Answer from the drawing. Dimensions are ordinates in mm from the lowest x, y and z of the part. Coordinates: 2 decimals unless noted, no trailing zeros. Write each loop counter-clockwise with the first axis right and the second up, starting at its lowest first coordinate (ties: lowest second). Pieces come first, ordered by that corner, then holes.
1) Each of these flat-tipped pins is pushed along its axis until it touches: pin 1 Ø1.6 at (y, z) = (1.5, 9.5) entering from -X; pin 2 Ø5 at (x, z) = (23, 21) entering from +Y; pin 3 Ø1 at (y, z) = (1.5, 8.5) entering from +X; pin 4 Ø0.6 at (x, y) = (45.5, 0.5) entering from -Z. Where does it stop, or does it pass through?
2) The part is cut by section A-A (z = 37). Determine the outline of the cut face in (x, y), then the cut area to 3 significant figures.
3) The part is cut by section C-C (y = 6). Determine the outline of the cut face in (x, z).
4) The part is cut by section B-B (x = 12.5). Determine the outline of the cut face in (y, z).
5) Find the intervals of material crossed by line 1 (Z direction, x = 6.5, y = 1.75); line 2 (Y direction, x = 50.5, z = 51), in increasing order.
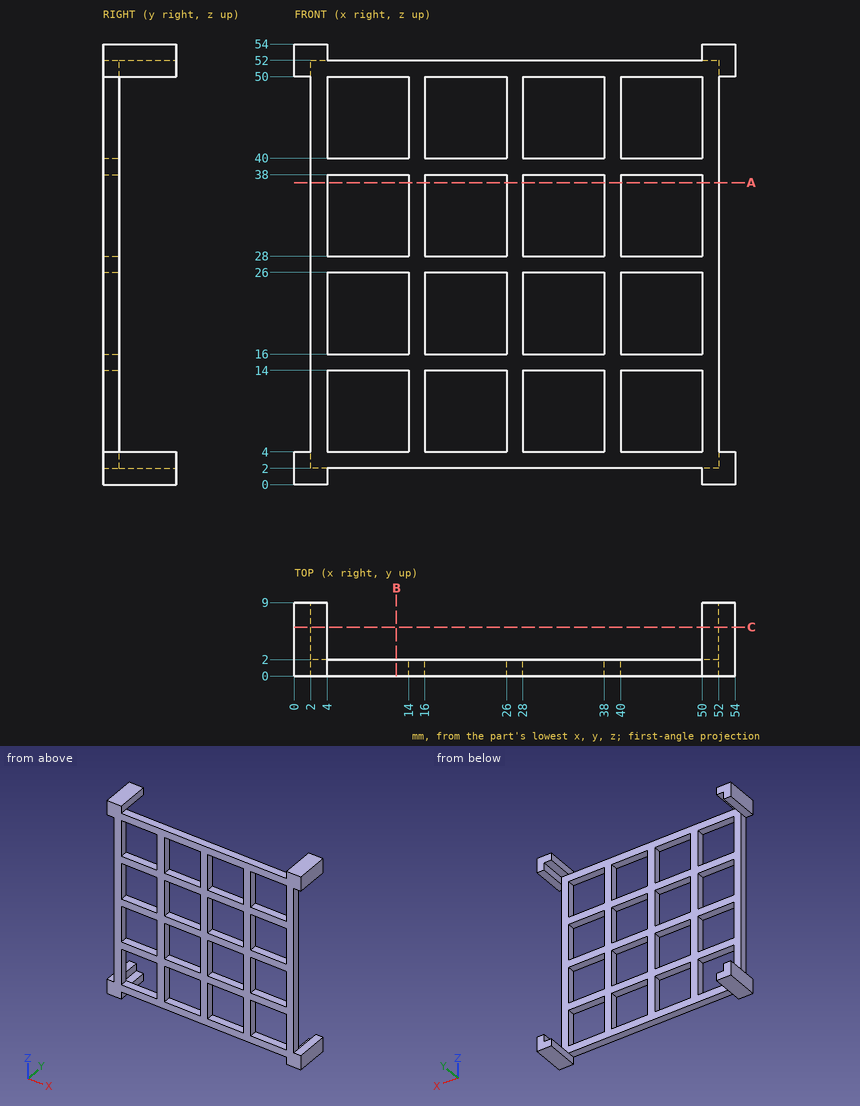
Reported:
1. pin 1: stops at x = 2
1. pin 2: passes through
1. pin 3: stops at x = 52
1. pin 4: stops at z = 2
2. outline: (2, 0) - (4, 0) - (4, 2) - (2, 2) - close; (14, 0) - (16, 0) - (16, 2) - (14, 2) - close; (26, 0) - (28, 0) - (28, 2) - (26, 2) - close; (38, 0) - (40, 0) - (40, 2) - (38, 2) - close; (50, 0) - (52, 0) - (52, 2) - (50, 2) - close
2. area: 20.0 mm2
3. outline: (0, 0) - (4, 0) - (4, 2) - (2, 2) - (2, 4) - (0, 4) - close; (0, 50) - (2, 50) - (2, 52) - (4, 52) - (4, 54) - (0, 54) - close; (50, 0) - (54, 0) - (54, 4) - (52, 4) - (52, 2) - (50, 2) - close; (50, 52) - (52, 52) - (52, 50) - (54, 50) - (54, 54) - (50, 54) - close
4. outline: (0, 2) - (2, 2) - (2, 4) - (0, 4) - close; (0, 14) - (2, 14) - (2, 16) - (0, 16) - close; (0, 26) - (2, 26) - (2, 28) - (0, 28) - close; (0, 38) - (2, 38) - (2, 40) - (0, 40) - close; (0, 50) - (2, 50) - (2, 52) - (0, 52) - close
5. line 1: z = 2 to 4, 14 to 16, 26 to 28, 38 to 40, 50 to 52
5. line 2: y = 0 to 2
